```python
from build123d import *

# Parameters (mm, degrees)
BOSS_EXTRUDE1_DEPTH     = 10
EXTRUDE_THIN1_DEPTH     = 10
CUT_EXTRUDE_THIN2_DEPTH = 10
BOSS_EXTRUDE2_DEPTH     = 10


# Read off the part's stored shape, not the designer's step: Extrude-Thin1
with BuildPart() as part:
    # Sketch1 → Boss-Extrude1 (new body)
    with BuildSketch(Plane(origin=(0, 0, 0), x_dir=(1, 0, 0), z_dir=(0, 1, 0))):
        with BuildLine():
            ThreePointArc((-17.640256265, -37.564229779), (0, 41.5), (17.640256265, -37.564229779))
            Line((17.640256265, -37.564229779), (19.765588345, -42.090040596))
            ThreePointArc((19.765588345, -42.090040596), (24.378319794, -39.597317132), (28.681103985, -36.601151269))
            Line((28.681103985, -36.601151269), (29.481767388, -35.626435952))
            Line((29.481767388, -35.626435952), (29.623728376, -35.842498756))
            ThreePointArc((29.623728376, -35.842498756), (-5.835552757, 46.132378261), (-19.765588345, -42.090040596))
            Line((-19.765588345, -42.090040596), (-17.640256265, -37.564229779))
        make_face()
    extrude(amount=BOSS_EXTRUDE1_DEPTH)

    # Extrude-Thin1 outline → Extrude-Thin1 (add)
    with BuildSketch(Plane(origin=(0, 0, 0), x_dir=(1, 0, 0), z_dir=(0, 1, 0))):
        with BuildLine():
            Line((-3, 50.921232979), (-1.25, 50.921232979))
            Line((-1.25, 50.921232979), (-1.25, 46.483195888))
            ThreePointArc((-1.25, 46.483195888), (0, 46.5), (1.25, 46.483195888))
            Line((1.25, 46.483195888), (1.25, 50.921232979))
            Line((1.25, 50.921232979), (3, 50.921232979))
            Line((3, 50.921232979), (3, 53.421232979))
            Line((3, 53.421232979), (-3, 53.421232979))
            Line((-3, 53.421232979), (-3, 50.921232979))
        make_face()
    extrude(amount=EXTRUDE_THIN1_DEPTH)

    # SurfaceCut1
    split(bisect_by=Plane(origin=(0, 0, 0), x_dir=(0, 0, -1), z_dir=(1, 0, 0)), keep=Keep.TOP)

    # Sketch3 → Cut-Extrude-Thin2 (cut)
    with BuildSketch(Plane(origin=(0, 0, 0), x_dir=(1, 0, 0), z_dir=(0, 1, 0))):
        Polygon((32.254075142, 30.132754798), (35.916621941, 33.795301597), (33.795301597, 35.916621941), (30.132754798, 32.254075142), align=None)
        Polygon((30.132754798, -32.254075142), (33.795301597, -35.916621941), (35.916621941, -33.795301597), (32.254075142, -30.132754798), align=None)
    extrude(amount=CUT_EXTRUDE_THIN2_DEPTH, mode=Mode.SUBTRACT)

    # Sketch1<6> → Boss-Extrude2 (add)
    with BuildSketch(Plane(origin=(0, 0, 0), x_dir=(1, 0, 0), z_dir=(0, 1, 0))):
        with BuildLine():
            Line((32.051958284, -39.538233554), (29.623728376, -35.842498756))
            ThreePointArc((29.623728376, -35.842498756), (29.15488394, -36.2248912), (28.681103985, -36.601151269))
            Line((28.681103985, -36.601151269), (31.765093661, -40.536758932))
            Line((31.765093661, -40.536758932), (33.437562335, -39.226192289))
            Line((33.437562335, -39.226192289), (33.162966722, -38.808261285))
            Line((33.162966722, -38.808261285), (32.051958284, -39.538233554))
        make_face()
        with BuildLine():
            ThreePointArc((28.681103985, -36.601151269), (29.15488394, -36.2248912), (29.623728376, -35.842498756))
            Line((29.623728376, -35.842498756), (29.481767388, -35.626435952))
            Line((29.481767388, -35.626435952), (28.681103985, -36.601151269))
        make_face()
    extrude(amount=BOSS_EXTRUDE2_DEPTH)


solid = part.part
```
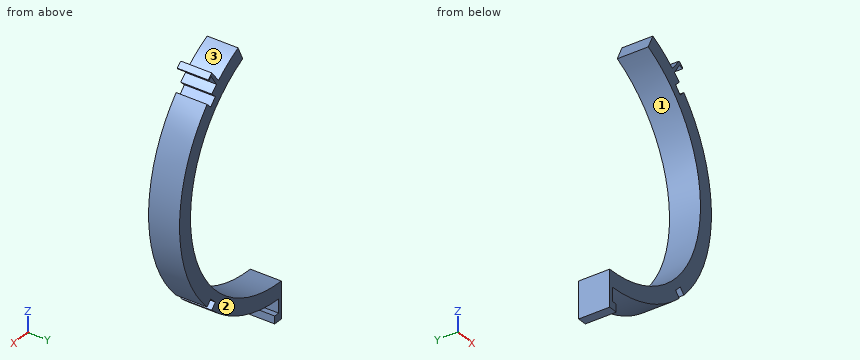
Verification items for the finished model (mm, model axes). Face numbers are marked on the shaded views. Round coordinates to 2 decimals unless told otherwise and drop trailing zeros. Write each loop counter-clockwise with the first axis right and the second up, starting at its lowest first coordinate (ties: lowest second). Pieces come first, ordered by that corner, then holes. Notation, with made-up numbers: (31, -16.5) - (90, -16.5) arc R24 cw to (90, 21.5) - close; hole circle Ø5 at (37.25, 39). An arc over 180 degrees is marked (long way). Answer as a JSON object with one key per item and string values. Group by question number.
Q1. Section check D-D, the plane x = 26.5. Enter the section's corners in (y, z), plus the area to 3 significant figures.
Q2. Section check A-A, the plane x = 38.5. Enter the section's corners in (y, z), plus the area to 3 significant figures.
Q3. Section check B-B, the plane y = 5.75. Enter the section's corners in (x, z).
Q4. Thickness scan on line 1 (Z direction, x = 31.5, y = 3.75); line 2 (Z direction, x = 30, y = 8.25); line 3 (Z direction, x = 34.5, y = 6.5). Record the ranges inside material, lowest first.
Q5. Mould release check, pull along X, two halves, no side actions. Record for the marked faces 1, 2 and 3: released by +X, released by -X, zero draft, split by the parting line, or undercut.
Q6. Go/stop test with flat-tipped pins: pin 1 Ø0.5 at (x, y) = (2.5, 3) entering from +Z; pin 2 Ø0.8 at (y, z) = (3.5, -52) entering from +X; pin 3 Ø1.3 at (y, z) = (6.5, -48) entering from +X. Record where each tip stops, or that it passes through.
Q7. Section check C-C, the plane z = 10. Enter the section's corners in (x, y), plus the area to 3 significant figures.
Found:
{
 "1": {"outline": "(0, -38.21) - (10, -38.21) - (10, -31.94) - (0, -31.94) - close; (0, 31.94) - (10, 31.94) - (10, 38.21) - (0, 38.21) - close", "area": "125 mm^2"},
 "2": {"outline": "(0, -26.08) - (10, -26.08) - (10, -15.49) - (0, -15.49) - close; (0, 15.49) - (10, 15.49) - (10, 26.08) - (0, 26.08) - close", "area": "212 mm^2"},
 "3": {"outline": "(0, -53.42) - (3, -53.42) - (3, -50.92) - (1.25, -50.92) - (1.25, -46.48) arc R46.5 ccw to (31.8, -33.92) - (30.13, -32.25) - (32.25, -30.13) - (33.92, -31.8) arc R46.5 ccw to (33.92, 31.8) - (32.25, 30.13) - (30.13, 32.25) - (31.8, 33.92) arc R46.5 ccw to (29.62, 35.84) - (32.05, 39.54) - (33.16, 38.81) - (33.44, 39.23) - (31.77, 40.54) - (28.68, 36.6) arc R46.5 ccw to (19.77, 42.09) - (17.64, 37.56) arc R41.5 cw to (0, -41.5) - close"},
 "4": {"line 1": "z = -34.21 to -33.62, -30.89 to -27.02, 27.02 to 30.89, 33.62 to 34.21, 38.7 to 40.2", "line 2": "z = -35.53 to -28.67, 28.67 to 35.53, 36.42 to 38.28", "line 3": "z = -31.18 to -23.07, 23.07 to 31.18"},
 "5": {"face 1": "released by -X", "face 2": "zero draft", "face 3": "undercut"},
 "6": {"pin 1": "stops at z = -41.41", "pin 2": "stops at x = 3", "pin 3": "stops at x = 1.25"},
 "7": {"outline": "(40.28, 0) - (45.41, 0) - (45.41, 10) - (40.28, 10) - close", "area": "51.3 mm^2"}
}
